from build123d import *

# Parameters (mm, degrees)
BOSS_EXTRUDE1_DEPTH    = 1.5
SKETCH2_W              = 41.5
SKETCH2_H              = 20.5
CUT_EXTRUDE1_DEPTH     = 1.5
F_12_0MM_DOWEL_HOLE1_D = 12


with BuildPart() as part:
    # Sketch1 → Boss-Extrude1 (new body)
    with BuildSketch(Plane.XY):
        with BuildLine():
            Line((50, 0), (310, 0))
            ThreePointArc((310, 0), (345.355339059, 14.644660941), (360, 50))
            Line((360, 50), (360, 310))
            ThreePointArc((360, 310), (345.355339059, 345.355339059), (310, 360))
            Line((310, 360), (50, 360))
            ThreePointArc((50, 360), (14.644660941, 345.355339059), (0, 310))
            Line((0, 310), (0, 50))
            ThreePointArc((0, 50), (14.644660941, 14.644660941), (50, 0))
        make_face()
    extrude(amount=BOSS_EXTRUDE1_DEPTH)

    # Sketch2 → Cut-Extrude1 (cut)
    with BuildSketch(Plane.XY.offset(1.5)):
        with Locations((54.25, 294.75)):
            Rectangle(SKETCH2_W, SKETCH2_H)
        with Locations((305.75, 294.75)):
            Rectangle(SKETCH2_W, SKETCH2_H)
        with Locations((305.75, 64.25)):
            Rectangle(SKETCH2_W, SKETCH2_H)
        with Locations((54.25, 64.25)):
            Rectangle(SKETCH2_W, SKETCH2_H)
    extrude(amount=-CUT_EXTRUDE1_DEPTH, mode=Mode.SUBTRACT)

    # Ø12.0mm Dowel Hole1 (through all)
    with Locations(Plane(origin=(92, 294.5, 1.5), x_dir=(1, 0, 0), z_dir=(0, 0, 1))):
        with Locations((0, 0), (176, 0), (176, -230), (0, -230)):
            Hole(F_12_0MM_DOWEL_HOLE1_D / 2)


solid = part.part
Here's how the part is built. I have some questions about the finished solid (model axes, mm). Round coordinates to 2 decimals unless told otherwise and drop trailing zeros. Order: outer loops, then holes, each group sorted by start corner. A loop starts at its lowest first (then second) coordinate and runs counter-clockwise, first axis right, second up. Notation, with made-up numbers: (52, -13) -> (106, -13) arc R25 ccw to (106, 0) -> close; hole circle Ø4 at (53, -39). An arc over 180 degrees is marked (long way). Use CSV: the item, a comma, the result in double quotes.
1. I want a section at A-A on y = 64.5. List the corners of the cut face in (x, z) for me, and give its area (4 significant figures).
Recorded:
outline,"(0, 0) -> (33.5, 0) -> (33.5, 1.5) -> (0, 1.5) -> close; (75, 0) -> (86, 0) -> (86, 1.5) -> (75, 1.5) -> close; (98, 0) -> (262, 0) -> (262, 1.5) -> (98, 1.5) -> close; (274, 0) -> (285, 0) -> (285, 1.5) -> (274, 1.5) -> close; (326.5, 0) -> (360, 0) -> (360, 1.5) -> (326.5, 1.5) -> close"
area,"379.5 mm2"
2. I need wall thicknesses on line 1 along X through (y, z) = (294.5, 1); line 2 along Y through (x, z) = (92, 0.75); line 3 along Y through (x, z) = (286.5, 1.4). Which ranges of each line are inside material? Lowest first, please.
Recorded:
line 1,"x = 0 to 33.5, 75 to 86, 98 to 262, 274 to 285, 326.5 to 360"
line 2,"y = 0 to 58.5, 70.5 to 288.5, 300.5 to 360"
line 3,"y = 0 to 54, 74.5 to 284.5, 305 to 360"
3. I want a section at B-B on x = 58.5. List the corners of the cut face in (y, z) for me, and give its area (4 significant figures).
Recorded:
outline,"(0, 0) -> (54, 0) -> (54, 1.5) -> (0, 1.5) -> close; (74.5, 0) -> (284.5, 0) -> (284.5, 1.5) -> (74.5, 1.5) -> close; (305, 0) -> (360, 0) -> (360, 1.5) -> (305, 1.5) -> close"
area,"478.5 mm2"
4. I want a section at C-C on z = 0.9. Give the number of separate pieces and of enclosed holes in the cut face, and give its area (3 significant figures).
Recorded:
separate pieces,"1"
enclosed holes,"8"
area,"124,000 mm2"
5. I'm going to push flat-ended pins straight in: P1, Ø14, axis at x = 92, y = 294.5, coming from the +Z side; P2, Ø0.8, axis at x = 311.5, z = 0.5, coming from the -Y side; P3, Ø11, axis at x = 268, y = 294.5, coming from the +Z side. Where does each tip first touch, or does it pass through?
Recorded:
P1,"stops at z = 1.5"
P2,"stops at y = 0.01"
P3,"passes through"
6. Thinking about a two-plate mould opening in X: for faces 1 (the face through (14.258, 15.036, 0.74)), 2 (the face through (92.78, 300.45, 0.74)), 3 (the face through (344.964, 14.258, 0.74)), which applies, pulls with the +X half, pulls with the -X half, needs draft (parallel to the pull), parting line crosses it, or undercut?
Recorded:
face 1,"pulls with the -X half"
face 2,"undercut"
face 3,"pulls with the +X half"
7. I want a section at D-D on x = 316.5. List the corners of the cut face in (y, z) for me, and give its area (3 significant figures).
Recorded:
outline,"(0.42, 0) -> (54, 0) -> (54, 1.5) -> (0.42, 1.5) -> close; (74.5, 0) -> (284.5, 0) -> (284.5, 1.5) -> (74.5, 1.5) -> close; (305, 0) -> (359.58, 0) -> (359.58, 1.5) -> (305, 1.5) -> close"
area,"477 mm2"
